For this review, take the finished solid that the model builds, in its own axes (mm). Face numbers are marked on the shaded views. A direction names the side the tool comes from. Coordinates: 2 decimals unless noted, no trailing zeros. Loops run counter-clockwise (first coordinate to the right, second up) from the corner with the lowest first, then second, coordinate; pieces in that order, holes last. Notation, with made-up numbers: M -6.5,-1 L 38.5,-1 A20 cw 38.5,14 Z; hole C 31.5,8.25 d10. An arc over 180 degrees is marked long. Answer as a JSON object with one key per item and string values. Group by question number.
Item 1: Add section B-B (x = 30.5). State the section outline as (y, z) points.
Item 2: Add section A-A (y = 35.5). State the section outline as (x, z) points.
Item 3: Insertion check: pin 1 (8 mm diameter, centred on y = -38, z = -4, fed in from +X); pin 2 (15 mm diameter, centred on x = -47, y = 42, fed in from +Z); pin 3 (4 mm diameter, centred on x = 42, z = -16, fed in from -Y). Each pin has a flat end and moves straight along its axis. Give the tip position at first contact, or say it passes through.
Item 4: Wall thickness on L1, parallel to Z at x = -57.5, y = 33; L2, parallel to Y at x = -36, z = -10; L3, parallel to Y at x = -38.5, z = -13: over which ranges is each line inside the solid? List them lowest first. Write a range as from..to.
Item 5: Tool access review of the marked faces 1, 2 and 3: name each direction out of +Z, -Z, +X, -X, +Y, -Y from which nothing blocks a thin tool from reaching the whole face with its end or side.
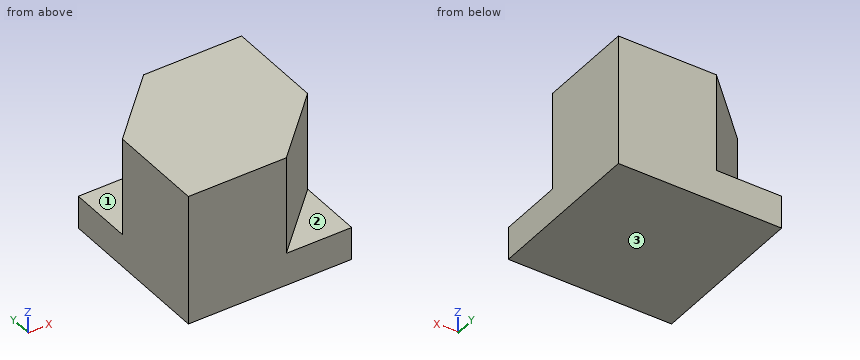
from build123d import *

# Parameters (mm, degrees)
F0_W     = 127
F0_H     = 101.6
F1_DEPTH = 63.5
F3_DEPTH = 76.2
F4_DEPTH = 76.2


with BuildPart() as f1:
    # F0 (on Front) → F1 (new body, symmetric)
    with BuildSketch(Plane.XZ):
        Rectangle(F0_W, F0_H)
    extrude(amount=F1_DEPTH, both=True)

    # F2 (on face) → F3 (cut)
    with BuildSketch(Plane.XY.offset(50.8)):
        Polygon((-12.7, 63.5), (-63.5, 63.5), (-63.5, 12.7), align=None)
    extrude(amount=-F3_DEPTH, mode=Mode.SUBTRACT)

    # F2 (on face) → F4 (cut)
    with BuildSketch(Plane.XY.offset(50.8)):
        Polygon((63.5, -63.5), (63.5, -12.7), (12.7, -63.5), align=None)
    extrude(amount=-F4_DEPTH, mode=Mode.SUBTRACT)


solid = f1.part
From the geometry:
{
 "1": {"outline": "M -63.5,-50.8 L 63.5,-50.8 L 63.5,50.8 L -45.7,50.8 L -45.7,-25.4 L -63.5,-25.4 Z"},
 "2": {"outline": "M -63.5,-50.8 L 63.5,-50.8 L 63.5,50.8 L -40.7,50.8 L -40.7,-25.4 L -63.5,-25.4 Z"},
 "3": {"pin 1": "stops at x = 42.2", "pin 2": "stops at z = -25.4", "pin 3": "stops at y = -36.2"},
 "4": {"L1": "z = -50.8..-25.4", "L2": "y = -63.5..40.2", "L3": "y = -63.5..37.7"},
 "5": {"face 1": "+Z, -X, +Y", "face 2": "+Z, +X, -Y", "face 3": "-Z, +X, -X, +Y, -Y"}
}
